from build123d import *

# Parameters (mm, degrees)
SKETCH2_R            = 2.5
BOSS_EXTRUDE2_DEPTH  = 15
SKETCH3_R            = 22.5
BOSS_EXTRUDE16_DEPTH = 39
BOSS_EXTRUDE22_START = -5
SKETCH3_4_R          = 22.5
BOSS_EXTRUDE22_DEPTH = 5
BOSS_EXTRUDE23_START = 6
SKETCH7_R            = 22.5
BOSS_EXTRUDE23_DEPTH = 6
SKETCH8_R            = 6
BOSS_EXTRUDE25_DEPTH = 30
SKETCH9_R            = 12
BOSS_EXTRUDE27_DEPTH = 5
SKETCH10_R           = 6
BOSS_EXTRUDE28_DEPTH = 110
SKETCH11_R           = 12
SKETCH11_R_2         = 0.5
BOSS_EXTRUDE30_DEPTH = 2


with BuildPart() as part:
    # Sketch2 → Boss-Extrude2 (new body)
    with BuildSketch(Plane(origin=(0, 0, 0), x_dir=(0, 0, -1), z_dir=(1, 0, 0))):
        with BuildLine():
            Line((-10, 64), (-15, 29))
            Line((-15, 29), (15, 29))
            Line((15, 29), (10, 64))
            ThreePointArc((10, 64), (0, 74), (-10, 64))
        make_face()
        with Locations((0, 64)):
            Circle(SKETCH2_R, mode=Mode.SUBTRACT)
    extrude(amount=BOSS_EXTRUDE2_DEPTH)

    # Sketch3 → Boss-Extrude16 (add)
    with BuildSketch(Plane(origin=(0, -10, 0), x_dir=(1, 0, 0), z_dir=(0, 1, 0))):
        with Locations(Location((7.5, 0, 0), (0, 0, 270))):
            Circle(SKETCH3_R)
    extrude(amount=BOSS_EXTRUDE16_DEPTH)

    # Sketch3<4> → Boss-Extrude22 (add)
    with BuildSketch(Plane(origin=(0, -10, 0), x_dir=(1, 0, 0), z_dir=(0, 1, 0)).offset(BOSS_EXTRUDE22_START)):
        with Locations(Location((7.5, 0, 0), (0, 0, 270))):
            Circle(SKETCH3_4_R)
    extrude(amount=BOSS_EXTRUDE22_DEPTH)

    # Sketch7 → Boss-Extrude23 (add)
    with BuildSketch(Plane.XZ.offset(15).offset(BOSS_EXTRUDE23_START)):
        with Locations(Location((7.5, 0, 0), (0, 0, 270))):
            Circle(SKETCH7_R)
    extrude(amount=-BOSS_EXTRUDE23_DEPTH)

    # Sketch8 → Boss-Extrude25 (add)
    with BuildSketch(Plane.XZ.offset(21)):
        with Locations(Location((7.5, 0, 0), (0, 0, 270))):
            Circle(SKETCH8_R)
    extrude(amount=BOSS_EXTRUDE25_DEPTH)

    # Sketch9 → Boss-Extrude27 (add)
    with BuildSketch(Plane.XZ.offset(51)):
        with Locations(Location((7.5, 0, 0), (0, 0, 270))):
            Circle(SKETCH9_R)
    extrude(amount=BOSS_EXTRUDE27_DEPTH)

    # Sketch10 → Boss-Extrude28 (add)
    with BuildSketch(Plane.XZ.offset(56)):
        with Locations(Location((7.5, 0, 0), (0, 0, 270))):
            Circle(SKETCH10_R)
    extrude(amount=BOSS_EXTRUDE28_DEPTH)

    # Sketch11 → Boss-Extrude30 (add)
    with BuildSketch(Plane.XZ.offset(166)):
        with Locations(Location((7.5, 0, 0), (0, 0, 270))):
            Circle(SKETCH11_R)
        with Locations(Location((7.5, 8, 0), (0, 0, 270))):
            Circle(SKETCH11_R_2, mode=Mode.SUBTRACT)
        with Locations(Location((2.797717982, 6.472135955, 0), (0, 0, 270))):
            Circle(SKETCH11_R_2, mode=Mode.SUBTRACT)
        with Locations(Location((-0.10845213, 2.472135955, 0), (0, 0, 270))):
            Circle(SKETCH11_R_2, mode=Mode.SUBTRACT)
        with Locations(Location((2.797717982, -6.472135955, 0), (0, 0, 270))):
            Circle(SKETCH11_R_2, mode=Mode.SUBTRACT)
        with Locations(Location((-0.10845213, -2.472135955, 0), (0, 0, 270))):
            Circle(SKETCH11_R_2, mode=Mode.SUBTRACT)
        with Locations(Location((7.5, -8, 0), (0, 0, 270))):
            Circle(SKETCH11_R_2, mode=Mode.SUBTRACT)
        with Locations(Location((12.202282018, -6.472135955, 0), (0, 0, 270))):
            Circle(SKETCH11_R_2, mode=Mode.SUBTRACT)
        with Locations(Location((15.10845213, -2.472135955, 0), (0, 0, 270))):
            Circle(SKETCH11_R_2, mode=Mode.SUBTRACT)
        with Locations(Location((15.10845213, 2.472135955, 0), (0, 0, 270))):
            Circle(SKETCH11_R_2, mode=Mode.SUBTRACT)
        with Locations(Location((12.202282018, 6.472135955, 0), (0, 0, 270))):
            Circle(SKETCH11_R_2, mode=Mode.SUBTRACT)
    extrude(amount=BOSS_EXTRUDE30_DEPTH)


solid = part.part
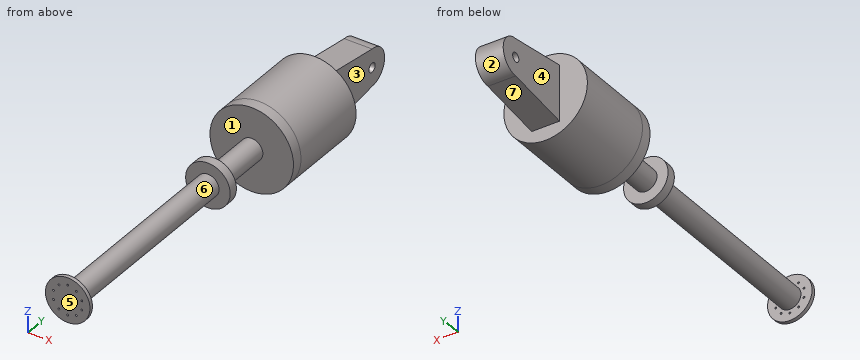
CAD build for the part. Positions are in the model's coordinates, mm. Face numbers are marked on the shaded views. A direction names the side the tool comes from. Give positions to 0.01 mm unless a question says otherwise; leave off trailing zeros. Write each loop counter-clockwise with the first axis right and the second up, starting at its lowest first coordinate (ties: lowest second). Pieces come first, ordered by that corner, then holes. Notation, with made-up numbers: (-18.5, -4) -> (32.5, -4) arc R16 cw to (32.5, 25) -> close; hole circle Ø4 at (48.5, 78). An arc over 180 degrees is marked (long way). Return JSON: item names as keys, results as strings.
Item 1: Drop flat-ended pins along their axis: pin 1 (10 mm diameter, centred on y = 4, z = 13.5, fed in from +X); pin 2 (4 mm diameter, centred on x = 24.5, z = -13.5, fed in from -Y); pin 3 (15 mm diameter, centred on y = 59.5, z = 0, fed in from +X). Give the stop position or say it passes through.
Answer below:
{"pin 1": "stops at x = 28.33", "pin 2": "stops at y = -21", "pin 3": "stops at x = 15"}
Item 2: Drill centre lines: probe 1 along Y at (x, z) = (16.5, -6); probe 2 along Y at (x, z) = (13.5, -8.5); probe 3 along Y at (x, z) = (28.5, -1). Where is each one in solid material? Low to high.
Answer below:
{"probe 1": "y = -168 to -166, -56 to -51, -21 to 29", "probe 2": "y = -168 to -166, -56 to -51, -21 to 69.27", "probe 3": "y = -21 to 29"}
Item 3: Two-plate mould, pull along Y, no slides. Class the marked faces 5, 6 and 7: +Y half, -Y half, draft (parallel to the pull), parting line (faces both ways), or undercut.
Answer below:
{"face 5": "-Y half", "face 6": "undercut", "face 7": "+Y half"}
Item 4: Band-saw the part on B-B (x = -11). List the corners of the cut face in (y, z), then the cut area to 3 significant figures.
Answer below:
{"outline": "(-21, -12.81) -> (29, -12.81) -> (29, 12.81) -> (-21, 12.81) -> close", "area": "1,280 mm2"}
Item 5: Band-saw the part on A-A (z = 18.5). List the corners of the cut face in (x, y).
Answer below:
{"outline": "(-5.31, -21) -> (20.31, -21) -> (20.31, 29) -> (-5.31, 29) -> close"}
Item 6: Tool access for the marked faces 1, 2, 3 and 4: list every direction of +Z, -Z, +X, -X, +Y, -Y with a clear straight run to the whole face (end or side of a thin tool).
Answer below:
{"face 1": "none", "face 2": "+X, -X, +Y", "face 3": "+Z, -Z, +X, +Y", "face 4": "+Z, -Z, -X, +Y"}
